The model under review builds one solid part; all positions refer to its coordinate system, in mm. Give positions to 0.01 mm unless a question says otherwise; leave off trailing zeros. Loops run counter-clockwise (first coordinate to the right, second up) from the corner with the lowest first, then second, coordinate; pieces in that order, holes last. Notation, with made-up numbers: (49, 67.25) - (53, 67.25) arc R24 cw to (53, 94.25) - close; hole circle Ø5 at (12, 28.5). An arc over 180 degrees is marked (long way). Return JSON: item names as keys, results as strings. Group by question number.
from build123d import *

# Parameters (mm, degrees)
BOSS_EXTRUDE1_DEPTH = 2.025
CUT_EXTRUDE1_REACH  = 6.05
SKETCH2_R           = 2.6


with BuildPart() as part:
    # Sketch1 → Boss-Extrude1 (new body, symmetric)
    with BuildSketch(Plane(origin=(0, 0, 0), x_dir=(1, 0, 0), z_dir=(0, 1, 0))):
        Polygon((4.742197554, 3.032995609), (-0.25555247, 5.623361356), (-4.997750023, 2.590365747), (-4.742197554, -3.032995609), (0.25555247, -5.623361356), (4.997750023, -2.590365747), align=None)
    extrude(amount=BOSS_EXTRUDE1_DEPTH, both=True)

    # Sketch2 → Cut-Extrude1 (cut, up to next)
    with BuildSketch(Plane(origin=(0, 2.025, 0), x_dir=(1, 0, 0), z_dir=(0, 1, 0)), mode=Mode.PRIVATE) as cut_extrude1_sk1:
        Circle(SKETCH2_R)
    cut_extrude1_tool1 = extrude(cut_extrude1_sk1.sketch, amount=-CUT_EXTRUDE1_REACH, mode=Mode.PRIVATE) & part.part
    add(cut_extrude1_tool1.solids().sort_by_distance((0, 2.025, 0))[0], mode=Mode.SUBTRACT)


solid = part.part
Item 1: Mouldability with a two-part tool opening along Z and no side actions: class faces 1 (the face through (2.59, 0.03, 4.13)), 2 (the face through (-1, 2.025, -3)), 3 (the face through (-2.59, 0.03, -4.13)), 4 (the face through (-0.338, 0.028, -2.578)) as +Z half, -Z half, draft (parallel to the pull), parting line (faces both ways), or undercut.
Item 2: For P1, Ø2, axis at x = 2.5, y = 1.5, coming from the -Z side; P2, Ø2, axis at x = 0.5, z = 1, coming from the +Y side; P3, Ø2, axis at x = -1, y = 0, coming from the -Z side, all flat-tipped, find the tip position at first contact; note any pin that passes through.
Item 3: Take a section at D-D (x = -4). State the section outline as (y, z) points (1 decimal), then the cut area to 3 significant figures.
Item 4: Take a section at B-B (x = 0.5). State the section outline as (y, z) points (3 decimals).
Item 5: For L1, parallel to X at y = 0.8, z = 0; L2, parallel to Z at x = -1, y = -1.1; L3, parallel to X at y = 1.6, z = 0.75, list the stretches that pass through material, from the lowest coordinate up. Write a range as from..to.
Item 6: Take a section at C-C (z = -2.25). State the section outline as (x, y) points (3 decimals).
Item 7: Take a section at A-A (y = -1.05). State the section outline as (x, z) points, then the cut area to 3 significant figures.
Check sheet entries:
{
 "1": {"face 1": "+Z half", "face 2": "draft", "face 3": "-Z half", "face 4": "undercut"},
 "2": {"P1": "stops at z = -4.71", "P2": "passes through", "P3": "stops at z = -5.62"},
 "3": {"outline": "(-2, -3.2) - (2, -3.2) - (2, 3.4) - (-2, 3.4) - close", "area": "26.9 mm^2"},
 "4": {"outline": "(-2.025, -5.232) - (2.025, -5.232) - (2.025, -2.551) - (-2.025, -2.551) - close; (-2.025, 2.551) - (2.025, 2.551) - (2.025, 5.467) - (-2.025, 5.467) - close"},
 "5": {"L1": "x = -4.88..-2.6, 2.6..4.88", "L2": "z = -5.15..-2.4, 2.4..4.97", "L3": "x = -4.85..-2.49, 2.49..4.91"},
 "6": {"outline": "(-4.982, -2.025) - (-1.303, -2.025) - (-1.303, 2.025) - (-4.982, 2.025) - close; (1.303, -2.025) - (4.778, -2.025) - (4.778, 2.025) - (1.303, 2.025) - close"},
 "7": {"outline": "(-5, -2.59) - (-0.26, -5.62) - (4.74, -3.03) - (5, 2.59) - (0.26, 5.62) - (-4.74, 3.03) - close; hole circle Ø5.2 at (0, 0)", "area": "61.1 mm^2"}
}
